Geometry: see drawing. Coordinates: mm, zero at the bounding-box minimum. Coordinates: 2 decimals unless noted, no trailing zeros. Loops run counter-clockwise (first coordinate to the right, second up) from the corner with the lowest first, then second, coordinate; pieces in that order, holes last. Notation, with made-up numbers: (60.25, -16.5) - (111.25, -16.5) arc R21 cw to (111.25, -10.5) - close; hole circle Ø6 at (89.5, 75). An arc over 180 degrees is marked (long way). Write item = value, one per line. Start each with the question number.
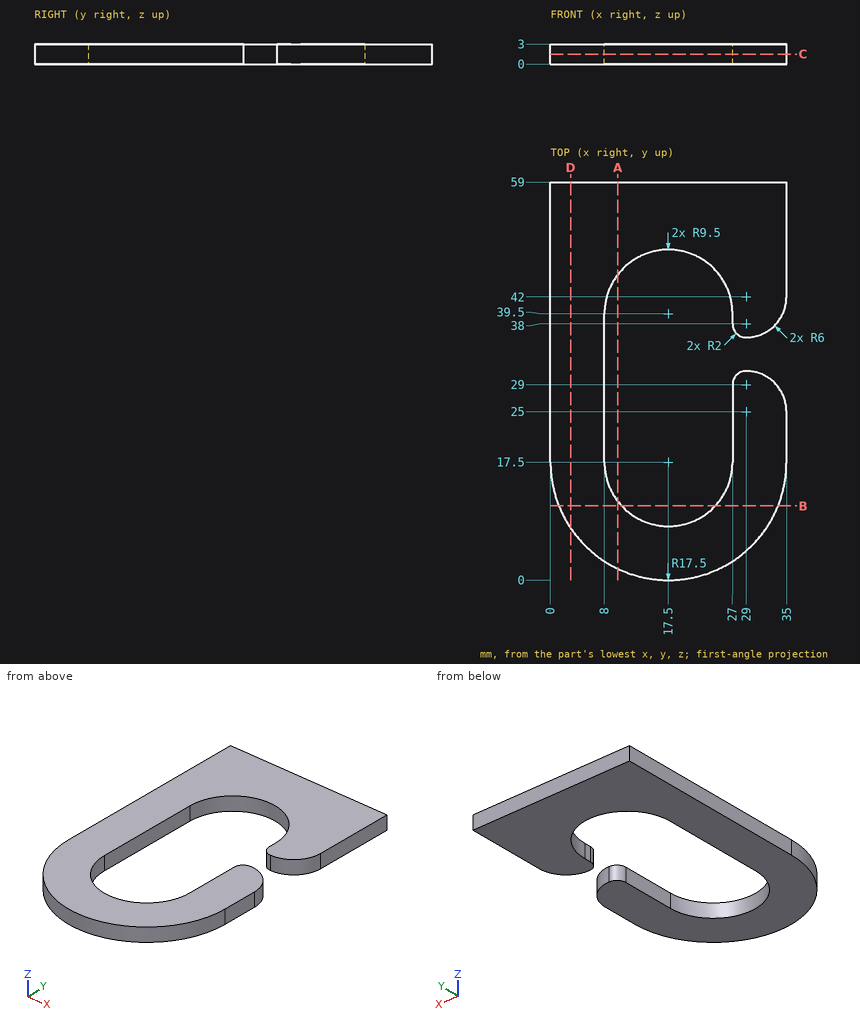
Item 1: Cut plane C-C (z = 1.5). Return the cut outline in (x, y).
Item 2: Cut plane D-D (x = 3). Return the cut outline in (y, z), then the cut area to 3 significant figures.
Item 3: Material intervals for L1, parallel to X at y = 24, z = 1.85; L2, parallel to X at y = 34, z = 2.7; L3, parallel to X at y = 11.5, z = 0.35, sorted ascending. Write a range as [from, to].
Item 4: Cut plane B-B (y = 11). Return the cut outline in (x, z), then the cut area to 3 significant figures.
Item 5: Cut plane A-A (x = 10). Return the cut outline in (y, z), then the cut area to 3 significant figures.
Responses:
q1.outline = (0, 17.5) arc R17.5 ccw to (35, 17.5) - (35, 25) arc R6 ccw to (29, 31) arc R2 ccw to (27, 29) - (27, 17.5) arc R9.5 cw to (8, 17.5) - (8, 39.5) arc R9.5 cw to (27, 39.5) - (27, 38) arc R2 ccw to (29, 36) arc R6 ccw to (35, 42) - (35, 59) - (0, 59) - close
q2.outline = (7.7, 0) - (59, 0) - (59, 3) - (7.7, 3) - close
q2.area = 154 mm2
q3.L1 = [0, 8], [27, 35]
q3.L2 = [0, 8]
q3.L3 = [1.06, 10.13], [24.87, 33.94]
q4.outline = (1.25, 0) - (10.57, 0) - (10.57, 3) - (1.25, 3) - close; (24.43, 0) - (33.75, 0) - (33.75, 3) - (24.43, 3) - close
q4.area = 55.9 mm2
q5.outline = (1.69, 0) - (11.67, 0) - (11.67, 3) - (1.69, 3) - close; (45.33, 0) - (59, 0) - (59, 3) - (45.33, 3) - close
q5.area = 70.9 mm2
